Verification items for the finished model (mm, model axes). Face numbers are marked on the shaded views. A direction names the side the tool comes from. Coordinates: 2 decimals unless noted, no trailing zeros. Order: outer loops, then holes, each group sorted by start corner. A loop starts at its lowest first (then second) coordinate and runs counter-clockwise, first axis right, second up. Notation, with made-up numbers: M 30.5,39 L 50.5,39 A21 ccw 50.5,52 Z; hole C 29.5,27 d9. An arc over 180 degrees is marked long. Use one line per item in the form item = value. Start each with the question number.
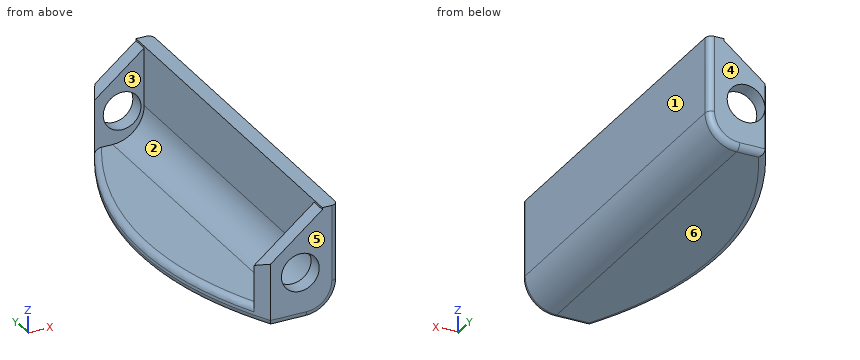
```python
from build123d import *

# Parameters (mm, degrees)
BOSS_EXTRUDE1_DEPTH = 144.78
RIB1_REACH          = 329.768
SKETCH3_WALL_W      = 771.836553366
SKETCH3_WALL_H      = 12.7
CUT_EXTRUDE1_DEPTH  = 289.56
FILLET1_R           = 5.08
SKETCH5_R           = 15.24
CUT_EXTRUDE2_DEPTH  = 328.768276772


with BuildPart() as part:
    # Sketch2 → Boss-Extrude1 (new, symmetric)
    with BuildSketch(Plane(origin=(0, 0, 0), x_dir=(1, 0, 0), z_dir=(0, 1, 0))):
        with BuildLine():
            Line((0, 0), (101.6, 0))
            ThreePointArc((101.6, 0), (119.560512242, -7.439487758), (127, -25.4))
            Line((127, -25.4), (127, -86.36))
            Line((127, -86.36), (114.3, -86.36))
            Line((114.3, -86.36), (114.3, -38.1))
            ThreePointArc((114.3, -38.1), (106.860512242, -20.139487758), (88.9, -12.7))
            Line((88.9, -12.7), (0, -12.7))
            Line((0, -12.7), (0, 0))
        make_face()
    extrude(amount=BOSS_EXTRUDE1_DEPTH, both=True)

    # Sketch3 wall → Rib1 (add, up to next)
    with BuildSketch(Plane(origin=(69.945945205, 144.78, 48.739427344), x_dir=(0.776098946536, 0, 0.630611152126), z_dir=(0.630611152126, 0, -0.776098946536)), mode=Mode.PRIVATE) as rib1_sk1:
        with Locations((0, 6.35)):
            Rectangle(SKETCH3_WALL_W, SKETCH3_WALL_H)
    rib1_tool1 = extrude(rib1_sk1.sketch, amount=RIB1_REACH, mode=Mode.PRIVATE) - part.part
    rib1 = rib1_tool1.solids().sort_by_distance((69.945945205, 144.78, 48.739427344))[0]
    add(rib1)

    # Mirror1: Rib1 across plane
    add(rib1.mirror(Plane.ZX))

    # Sketch4 → Cut-Extrude1 (cut)
    with BuildSketch(Plane(origin=(0, 0, 0), x_dir=(-1, 0, 0), z_dir=(0, 0, -1))):
        with BuildLine():
            Line((-81.089693515, 144.78), (0, 144.78))
            Line((0, 144.78), (0, -144.78))
            Line((0, -144.78), (-72.453889421, -144.78))
            add(Edge.make_bspline(
                [(-81.089693515, 144.78), (-22.496571769, 42.315365933), (-25.923555625, -60.216187191), (-72.453889421, -144.78)],
                knots=[0, 0, 0, 0, 1, 1, 1, 1], degree=3))
        make_face()
    extrude(amount=-CUT_EXTRUDE1_DEPTH, mode=Mode.SUBTRACT)

    # Fillet1
    fillet1_edges = [part.edges().sort_by_distance(p)[0] for p in [
        (127, 144.78, 55.88),
        (119.560512242, 144.78, 7.439487758),
        (91.344846758, 144.78, 0),
        (127, -144.78, 55.88),
        (119.560512242, -144.78, 7.439487758),
        (37.55873854, 0.944564154, 0),
        (87.02694471, -144.78, 0),
        (37.555382274, 0.862578583, 12.7),
    ]]
    fillet(fillet1_edges, radius=FILLET1_R)

    # Sketch5 → Cut-Extrude2 (cut, through all)
    with BuildSketch(Plane.XZ.offset(144.78)):
        with Locations(Location((96.52, 38.1, 0), (0, 0, 270))):
            Circle(SKETCH5_R)
    extrude(amount=-CUT_EXTRUDE2_DEPTH, mode=Mode.SUBTRACT)


solid = part.part
```
1. Depth check by flat-ended pin: P1, Ø4, axis at x = 96.5, y = -101.5, coming from the +Z side; P2, Ø10, axis at y = -62, z = 17.5, coming from the +X side; P3, Ø2, axis at x = 68, z = 36.5, coming from the +Y side; P4, Ø24.5, axis at x = 96.52, z = 38.1, coming from the -Y side. Enter the tip coordinate at first touch or a pass-through.
2. Cross-section at B-B on z = 65. Enter the section's corners in (x, y), and give its area (3 significant figures).
3. Release check for a two-part mould opening along Y. For the marked faces 3, 4, 5 and 6 record: pulls with the +Y half, pulls with the -Y half, needs draft (parallel to the pull), parting line crosses it, or undercut.
4. Tool access check on the marked faces 1 and 2. Record the directions out of +Z, -Z, +X, -X, +Y, -Y that give a thin tool (end or side, any length) a straight path to the whole face; none if there is none.
5. Material ranges on line 1 along Y through (x, z) = (107, 70); line 2 along X through (y, z) = (108, 79); line 3 along Z through (x, y) = (77, 16), recorded low to high.
6. Cross-section at A-A on x = 96.52. Enter the section's corners in (y, z), and give its area (3 significant figures).
Final values:
q1.P1 = 14.58
q1.P2 = 126.83
q1.P3 = -132.08
q1.P4 = through
q2.outline = M 89.96,-144.78 L 121.92,-144.78 A5.08 ccw 127,-139.7 L 127,139.7 A5.08 ccw 121.92,144.78 L 89.96,144.78 L 89.96,132.08 L 114.3,132.08 L 114.3,-132.08 L 89.96,-132.08 Z
q2.area = 4,280 mm2
q3.face_3 = undercut
q3.face_4 = pulls with the +Y half
q3.face_5 = pulls with the -Y half
q3.face_6 = needs draft
q4.face_1 = +Z, -Z, +X, +Y, -Y
q4.face_2 = +Z, -X
q5.line_1 = -144.78 to -132.08, 132.08 to 144.78
q5.line_2 = 114.3 to 127
q5.line_3 = 0 to 12.7
q6.outline = M -144.78,5.08 A5.08 ccw -139.7,0 L 139.7,0 A5.08 ccw 144.78,5.08 L 144.78,22.86 L 132.08,22.86 L 132.08,13.87 L -132.08,13.87 L -132.08,22.86 L -144.78,22.86 Z; M -144.78,53.34 L -132.08,53.34 L -132.08,70.33 L -144.78,70.33 Z; M 132.08,53.34 L 144.78,53.34 L 144.78,70.33 L 132.08,70.33 Z
q6.area = 4,670 mm2
